```python
from build123d import *

# Parameters (mm, degrees)
SKETCH1_R                    = 1.525
SKETCH1_R_2                  = 6.5
SKETCH1_R_3                  = 1.5
BOSS_EXTRUDE1_DEPTH          = 3
CSK_FOR_M3_SFHCS1_AT_2_COUNT = 2
CSK_FOR_M3_SFHCS1_AT_2_PITCH = 136.5
CSK_FOR_M3_SFHCS1_AT_3_COUNT = 2
CSK_FOR_M3_SFHCS1_AT_3_PITCH = 155.125562046
CSK_FOR_M3_SFHCS1_AT_4_COUNT = 2
CSK_FOR_M3_SFHCS1_AT_4_PITCH = 73.7


with BuildPart() as part:
    # Sketch1 → Boss-Extrude1 (new body)
    with BuildSketch(Plane(origin=(0, 0, 0), x_dir=(0, 0, -1), z_dir=(1, 0, 0))):
        with BuildLine():
            Line((-71.5, 41.1), (71.5, 41.1))
            ThreePointArc((71.5, 41.1), (72.207106781, 40.807106781), (72.5, 40.1))
            Line((72.5, 40.1), (72.5, -40.1))
            ThreePointArc((72.5, -40.1), (72.207106781, -40.807106781), (71.5, -41.1))
            Line((71.5, -41.1), (-71.5, -41.1))
            ThreePointArc((-71.5, -41.1), (-72.207106781, -40.807106781), (-72.5, -40.1))
            Line((-72.5, -40.1), (-72.5, 40.1))
            ThreePointArc((-72.5, 40.1), (-72.207106781, 40.807106781), (-71.5, 41.1))
        make_face()
        with Locations((26.5, -15.6)):
            Circle(SKETCH1_R, mode=Mode.SUBTRACT)
        with Locations(Location((62.5, -15.6, 0), (0, 0, 180))):
            Circle(SKETCH1_R, mode=Mode.SUBTRACT)
        with Locations((22.5, 21.1)):
            Circle(SKETCH1_R_2, mode=Mode.SUBTRACT)
        with Locations((7.5, 21.1)):
            Circle(SKETCH1_R_3, mode=Mode.SUBTRACT)
        with Locations(Location((57.5, 21.1, 0), (0, 0, 180))):
            Circle(SKETCH1_R_3, mode=Mode.SUBTRACT)
        with Locations(Location((42.5, 21.1, 0), (0, 0, 180))):
            Circle(SKETCH1_R_2, mode=Mode.SUBTRACT)
        with BuildLine():
            Line((33, -0.1), (56, -0.1))
            ThreePointArc((56, -0.1), (57.414213562, -0.685786438), (58, -2.1))
            Line((58, -2.1), (58, -29.1))
            ThreePointArc((58, -29.1), (57.414213562, -30.514213562), (56, -31.1))
            Line((56, -31.1), (33, -31.1))
            ThreePointArc((33, -31.1), (31.585786438, -30.514213562), (31, -29.1))
            Line((31, -29.1), (31, -2.1))
            ThreePointArc((31, -2.1), (31.585786438, -0.685786438), (33, -0.1))
        make_face(mode=Mode.SUBTRACT)
    extrude(amount=BOSS_EXTRUDE1_DEPTH)

    # Sketch3 → CSK for M3 SFHCS1 (revolve, cut)
    with BuildSketch(Plane(origin=(3, 36.85, 68.25), x_dir=(0, 0, -1), z_dir=(0, 1, 0))):
        Polygon((0, 0), (0, 3), (1.7, 3), (1.7, 1.66), (3.36, 0), align=None)
    csk_for_m3_sfhcs1 = revolve(axis=Axis((9.35, 36.85, 68.25), (-1, 0, 0)), mode=Mode.SUBTRACT)

    # CSK for M3 SFHCS1 at 2: CSK for M3 SFHCS1 ×2
    with Locations(*[(0, 0, -i * CSK_FOR_M3_SFHCS1_AT_2_PITCH) for i in range(1, CSK_FOR_M3_SFHCS1_AT_2_COUNT)]):
        add(csk_for_m3_sfhcs1, mode=Mode.SUBTRACT)

    # CSK for M3 SFHCS1 at 3: CSK for M3 SFHCS1 ×2
    with Locations(*[Vector(0, -0.4750990038526292, -0.8799323477053447) * (i * CSK_FOR_M3_SFHCS1_AT_3_PITCH) for i in range(1, CSK_FOR_M3_SFHCS1_AT_3_COUNT)]):
        add(csk_for_m3_sfhcs1, mode=Mode.SUBTRACT)

    # CSK for M3 SFHCS1 at 4: CSK for M3 SFHCS1 ×2
    with Locations(*[(0, -i * CSK_FOR_M3_SFHCS1_AT_4_PITCH, 0) for i in range(1, CSK_FOR_M3_SFHCS1_AT_4_COUNT)]):
        add(csk_for_m3_sfhcs1, mode=Mode.SUBTRACT)


solid = part.part
```
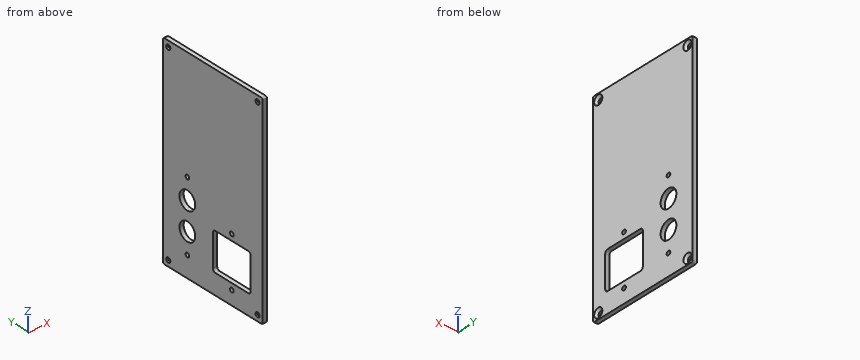
Input: part model. Units: mm. Frame: model coordinates. Give positions to 0.01 mm unless a question says otherwise; leave off trailing zeros. Order: outer loops, then holes, each group sorted by start corner. A loop starts at its lowest first (then second) coordinate and runs counter-clockwise, first axis right, second up. Notation, with made-up numbers: M 36,8.5 L 56,8.5 A20 ccw 56,21.5 Z; hole C 60,63 d4. An arc over 180 degrees is marked long. One line per question, with ' | ' between items.
1) Ray query, L1, parallel to Y at x = 2, z = -42.5; L2, parallel to Z at x = 1.05, y = -36.85; L3, parallel to Y at x = 0.35, z = 68.25. Return the intervals inside material, ascending.
Filled in:
L1: y = -41.1 to -31.1, -0.1 to 14.6, 27.6 to 41.1 | L2: z = -72.5 to -69.95, -66.55 to 66.55, 69.95 to 72.5 | L3: y = -41.1 to -38.55, -35.15 to 35.15, 38.55 to 41.1
2) Contact query for a flat-ended pin moving along its axis: P1, Ø10.5, axis at y = 21.1, z = -42.5, coming from the +X side. Output: stop coordinate, or through.
Filled in:
P1: passes through
3) Section A-A on z = -42.5. Output: boundary loops of the cut face in (x, y), and give its area (3 significant figures).
Filled in:
outline: M 0,-41.1 L 3,-41.1 L 3,-31.1 L 0,-31.1 Z; M 0,-0.1 L 3,-0.1 L 3,14.6 L 0,14.6 Z; M 0,27.6 L 3,27.6 L 3,41.1 L 0,41.1 Z | area: 115 mm2
4) Section D-D on z = -22.5. Output: boundary loops of the cut face in (x, y).
Filled in:
outline: M 0,-41.1 L 3,-41.1 L 3,14.6 L 0,14.6 Z; M 0,27.6 L 3,27.6 L 3,41.1 L 0,41.1 Z
5) Section C-C on x = 2.3. State how many separate pieces and enclosed holes the cut face has, and give its area (3 significant figures).
Filled in:
separate pieces: 1 | enclosed holes: 11 | area: 10,700 mm2
6) Section B-B on y = -36.85. Output: boundary loops of the cut face in (x, z), and give its area (3 significant figures).
Filled in:
outline: M 0,-72.5 L 3,-72.5 L 3,-71.61 L 1.34,-69.95 L 0,-69.95 Z; M 0,-66.55 L 1.34,-66.55 L 3,-64.89 L 3,64.89 L 1.34,66.55 L 0,66.55 Z; M 0,69.95 L 1.34,69.95 L 3,71.61 L 3,72.5 L 0,72.5 Z | area: 409 mm2
